Part model, mm, in its own coordinate system. Give positions to 0.01 mm unless a question says otherwise; leave off trailing zeros. Order: outer loops, then holes, each group sorted by start corner. A loop starts at its lowest first (then second) coordinate and runs counter-clockwise, first axis right, second up. Notation, with made-up numbers: M -10,31.25 L 40,31.25 A24 ccw 40,41.25 Z; hole C 65,46 d9. An arc over 180 degrees is marked long. Return JSON: item names as keys, results as strings.
Autodesk Inventor part; units mm, degrees
ref_plane "YZ Plane" through (0, 0, 0) normal (1, 0, 0) x (0, 1, 0)
ref_plane "XZ Plane" through (0, 0, 0) normal (0, 1, 0) x (-1, 0, 0)
ref_plane "XY Plane" through (0, 0, 0) normal (0, 0, 1) x (1, 0, 0)
sketch "Эскиз1" plane through (0, 0, 0) normal (0, 1, 0) x (-1, 0, 0)
  line L0 (0, 0) -> (3, 0)
  line L1 (3, 0) -> (3, -40)
  line L2 (3, -40) -> (0, -40)
  line L3 (0, -40) -> (0, 0)
  line L4 (0, 0) -> (1, 0)
  line L5 (0, -5) -> (0, 0)
  line L6 (3, -40) -> (2, -40)
  line L7 (3, -35) -> (3, -40)
  dimension "d0" = 40
  dimension "d1" = 3
extrude "Выдавливание1" add sketch "Эскиз1" along normal blind 6
sketch "Эскиз2" plane through (0, 0, 0) normal (0, -1, 0) x (1, 0, 0)
  line L0 (-3, 0) -> (0, 0)
  line L1 (-3, 0) -> (-2, 0)
  line L2 (-2, -5) -> (-1, -5)
  line L3 (-1, -5) -> (-1, -35)
  line L4 (-1, -35) -> (-2, -35)
  line L5 (-2, -35) -> (-2, -5)
  point P0 (0, -40)
  dimension "d13" = 30
  dimension "d14" = 1
extrude "Выдавливание2" add sketch "Эскиз2" along normal blind 1
fillet "Сопряжение1" radius 1 4 edges at (0, 3, 0) (-3, 3, 0) (0, 3, -40) (-3, 3, -40)
fillet "Сопряжение2" radius 0.3 4 edges at (-1, -0.5, -35) (-2, -0.5, -35) (-1, -0.5, -5) (-2, -0.5, -5)
sketch "Эскиз3" plane through (0, 6, 0) normal (0, 1, 0) x (1, 0, 0)
  line L0 (0, 0) -> (-1.5, 0)
  line L1 (0, 1) -> (0, 39)
  line L2 (0, 20) -> (0, 30)
  circle A0 centre (-1.5, 10) radius 1.1
  circle A1 centre (-1.5, 20) radius 1.1
  circle A2 centre (-1.5, 30) radius 1.1
  dimension "d23" = 2.2
  dimension "d24" = 2.2
  dimension "d25" = 2.2
extrude "Выдавливание3" cut sketch "Эскиз3" against normal blind 4
properties part number "Bush" material "Медь"
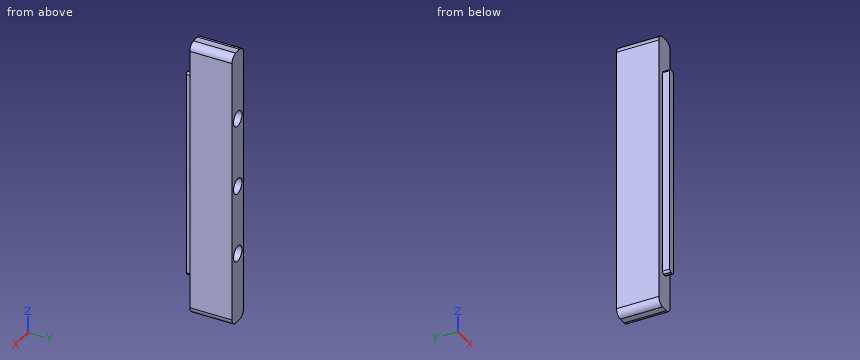
Q1. Pin check, flat tips, straight feed: pin 1 (1.1 mm diameter, centred on x = -1.5, z = -9.5, fed in from +Y); pin 2 (0.8 mm diameter, centred on y = -0.5, z = -23, fed in from +X); pin 3 (0.5 mm diameter, centred on y = -0.5, z = -23, fed in from -X). Stop position of each tip, or through.
Established:
{"pin 1": "stops at y = 2", "pin 2": "stops at x = -1", "pin 3": "stops at x = -2"}
Q2. Band-saw the part on B-B (y = 5.25). Give the cut face in (x, z).
Established:
{"outline": "M -3,-39 A1 ccw -2,-40 L -1,-40 A1 ccw 0,-39 L 0,-1 A1 ccw -1,0 L -2,0 A1 ccw -3,-1 Z; hole C -1.5,-30 d2.2; hole C -1.5,-20 d2.2; hole C -1.5,-10 d2.2"}
Q3. Band-saw the part on C-C (z = -30). Give the cut face in (x, y).
Established:
{"outline": "M -3,0 L -2,0 L -2,-1 L -1,-1 L -1,0 L 0,0 L 0,6 L -0.4,6 L -0.4,2 L -2.6,2 L -2.6,6 L -3,6 Z"}
Q4. Probe line 1 along Z through (x, y) = (-1.5, 4.7); line 2 along Z through (x, y) = (-2.45, 2.25); line 3 along X through (y, z) = (3.45, -20). List the from-to ranges inside material, lowest first.
Established:
{"line 1": "z = -40 to -31.1, -28.9 to -21.1, -18.9 to -11.1, -8.9 to 0", "line 2": "z = -39.89 to -30.55, -29.45 to -20.55, -19.45 to -10.55, -9.45 to -0.11", "line 3": "x = -3 to -2.6, -0.4 to 0"}
Q5. Band-saw the part on A-A (z = -12.5). Give the cut face in (x, y).
Established:
{"outline": "M -3,0 L -2,0 L -2,-1 L -1,-1 L -1,0 L 0,0 L 0,6 L -3,6 Z"}
